Here's how the part is built. I have some questions about the finished solid (model axes, mm). Face numbers are marked on the shaded views. Round coordinates to 2 decimals unless told otherwise and drop trailing zeros. Loops run counter-clockwise (first coordinate to the right, second up) from the corner with the lowest first, then second, coordinate; pieces in that order, holes last. Notation, with made-up numbers: (46.25, -8) -> (79.25, -8) arc R20 ccw to (79.25, 8) -> close; hole circle Ø9 at (42, 89.25). An arc over 180 degrees is marked (long way). One line per item, written item: value. Start each with the question number.
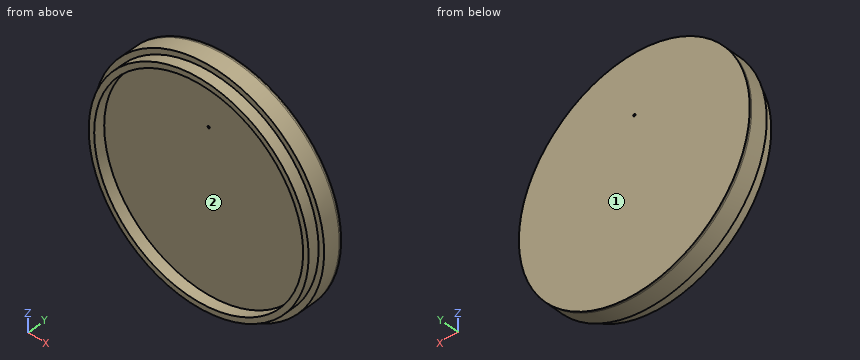
```python
from build123d import *

# Parameters (mm, degrees)
F0_R     = 50
F1_DEPTH = 13
F2_T     = -2.5
F3_R     = 52.5
F3_R_2   = 0.5
F4_DEPTH = 8
F5_DEPTH = 0.5


with BuildPart() as f1:
    # F0 (on Front) → F1 (new body)
    with BuildSketch(Plane.XZ):
        Circle(F0_R)
    extrude(amount=F1_DEPTH)

    # F2
    f2_openings = [f1.faces().sort_by_distance(p)[0] for p in [
        (0, -13, 0),
    ]]
    offset(amount=F2_T, openings=f2_openings)

    # F3 (on Front) → F4 (join)
    with BuildSketch(Plane.XZ):
        Circle(F3_R)
        with Locations((0, 25.5)):
            Circle(F3_R_2, mode=Mode.SUBTRACT)
    extrude(amount=F4_DEPTH)

    # F3 (on Front) → F5 (join, symmetric)
    with BuildSketch(Plane.XZ):
        Circle(F3_R)
        with Locations((0, 25.5)):
            Circle(F3_R_2, mode=Mode.SUBTRACT)
    extrude(amount=F5_DEPTH, both=True)


solid = f1.part
```
Q1. I want a section at A-A on z = 0. Please give me the cut outline in (x, y), plus the area to 4 significant figures.
Q2. Will these pins go through, and if not, where does the flat tip stop? P1, Ø6, axis at x = -40.5, y = -10.5, coming from the -Z side; P2, Ø0.8, axis at x = 0, z = 25.5, coming from the -Y side; P3, Ø3, axis at y = -6, z = -38, coming from the -X side.
Q3. If I drill on line 1 along Z through (x, y) = (0, -6.3); line 2 along Y through (x, z) = (16, -12); line 3 along X through (y, z) = (-12, -4), over which ranges is the centre line in solid material (lowest first)?
Q4. I want a section at B-B on y = -9.25. Please give me the cut outline in (x, z), plus the area to 3 significant figures.
Q5. I want a section at C-C on x = 5. Please give me the cut outline in (y, z), plus the area to 3 significant figures.
Q6. If we mould it in two halves opening along X, with no side actions, what happens to the marked faces 1 and 2? For each: released by +X, released by -X, zero draft, split by the parting line, or undercut.
Answers below:
1. outline: (-52.5, -8) -> (-50, -8) -> (-50, -13) -> (-47.5, -13) -> (-47.5, -8) -> (47.5, -8) -> (47.5, -13) -> (50, -13) -> (50, -8) -> (52.5, -8) -> (52.5, 0.5) -> (-52.5, 0.5) -> close
1. area: 917.5 mm^2
2. P1: stops at z = -35.32
2. P2: stops at y = -2.5
2. P3: stops at x = -37.74
3. line 1: z = -52.5 to 25, 26 to 52.5
3. line 2: y = -8 to 0.5
3. line 3: x = -49.84 to -47.33, 47.33 to 49.84
4. outline: circle Ø100 at (0, 0); hole circle Ø95 at (0, 0)
4. area: 766 mm^2
5. outline: (-13, -49.75) -> (-8, -49.75) -> (-8, -52.26) -> (0.5, -52.26) -> (0.5, 52.26) -> (-8, 52.26) -> (-8, 49.75) -> (-13, 49.75) -> (-13, 47.24) -> (-8, 47.24) -> (-8, -47.24) -> (-13, -47.24) -> close
5. area: 914 mm^2
6. face 1: zero draft
6. face 2: undercut
